Source: CAD feature listing. Evaluate the final solid. Frame: model axes, mm. Face numbers are marked on the shaded views. A direction names the side the tool comes from. Give positions to 0.01 mm unless a question says otherwise; leave off trailing zeros. Loops run counter-clockwise (first coordinate to the right, second up) from the corner with the lowest first, then second, coordinate; pieces in that order, holes last. Notation, with made-up numbers: M 75.25,23 L 120.25,23 A22 ccw 120.25,43 Z; hole C -38,89 d11. An arc over 180 degrees is marked long. Answer in a Markdown table with one row per item.
```python
from build123d import *

# Parameters (mm, degrees)
SKETCH2_W             = 20.32
SKETCH2_H             = 7.62
SKETCH2_R             = 1.905
BOSS_EXTRUDE1_DEPTH   = 12.7
BOSS_EXTRUDE1_2_DEPTH = 12.7
SKETCH4_W             = 3.81
SKETCH4_H             = 55.88
BOSS_EXTRUDE2_DEPTH   = 28.702
SKETCH5_W             = 27.94
SKETCH5_H             = 55.88
BOSS_EXTRUDE3_DEPTH   = 7.62
SKETCH6_R             = 10.922
BOSS_EXTRUDE6_DEPTH   = 55.88
SKETCH10_W            = 20.32
SKETCH10_H            = 16.002
BOSS_EXTRUDE7_DEPTH   = 7.62
SKETCH11_W            = 20.32
SKETCH11_H            = 16.002
BOSS_EXTRUDE8_DEPTH   = 7.62
SKETCH12_R            = 10.922
BOSS_EXTRUDE9_DEPTH   = 19.05
SKETCH14_R            = 2.921
BOSS_EXTRUDE10_DEPTH  = 74.93
SKETCH17_R            = 5.08
CUT_EXTRUDE3_DEPTH    = 32.766
SKETCH18_W            = 6.35
SKETCH18_H            = 7.62
CUT_EXTRUDE4_DEPTH    = 28.702


with BuildPart() as part:
    # Sketch2 → Boss-Extrude1 (new body)
    with BuildSketch(Plane.XY):
        with Locations((0, 24.13)):
            Rectangle(SKETCH2_W, SKETCH2_H)
        with Locations((4.699, 24.13)):
            Circle(SKETCH2_R, mode=Mode.SUBTRACT)
        with Locations((-4.699, 24.13)):
            Circle(SKETCH2_R, mode=Mode.SUBTRACT)
    extrude(amount=BOSS_EXTRUDE1_DEPTH)



with BuildPart() as body_2:
    # Sketch2 → Boss-Extrude1 2 (new body)
    with BuildSketch(Plane.XY):
        with Locations((0, -24.13)):
            Rectangle(SKETCH2_W, SKETCH2_H)
        with Locations((-4.699, -24.13)):
            Circle(SKETCH2_R, mode=Mode.SUBTRACT)
        with Locations((4.699, -24.13)):
            Circle(SKETCH2_R, mode=Mode.SUBTRACT)
    extrude(amount=BOSS_EXTRUDE1_2_DEPTH)


with BuildPart() as part_1:
    add(part.part)

    add(body_2.part)  # Boss-Extrude2 merges body 2
    # Sketch4 → Boss-Extrude2 (add)
    with BuildSketch(Plane.XY.offset(12.7)):
        with Locations((-12.065, 0)):
            Rectangle(SKETCH4_W, SKETCH4_H)
        with Locations((12.065, 0)):
            Rectangle(SKETCH4_W, SKETCH4_H)
    extrude(amount=-BOSS_EXTRUDE2_DEPTH)

    # Sketch5 → Boss-Extrude3 (add)
    with BuildSketch(Plane(origin=(0, 0, -16.002), x_dir=(-1, 0, 0), z_dir=(0, 0, -1))):
        Rectangle(SKETCH5_W, SKETCH5_H)
    extrude(amount=BOSS_EXTRUDE3_DEPTH)

    # Sketch6 → Boss-Extrude6 (add)
    with BuildSketch(Plane(origin=(0, 27.94, 0), x_dir=(1, 0, 0), z_dir=(0, 1, 0))):
        with BuildLine():
            Line((8.710385525, 23.622), (13.97, 23.622))
            Line((13.97, 23.622), (13.97, 34.544))
            ThreePointArc((13.97, 34.544), (0, 48.514), (-13.97, 34.544))
            Line((-13.97, 34.544), (-13.97, 23.622))
            Line((-13.97, 23.622), (-8.710385525, 23.622))
            ThreePointArc((-8.710385525, 23.622), (0, 20.574), (8.710385525, 23.622))
        make_face()
        with Locations((0, 34.544)):
            Circle(SKETCH6_R, mode=Mode.SUBTRACT)
    extrude(amount=-BOSS_EXTRUDE6_DEPTH)

    # Sketch10 → Boss-Extrude7 (add)
    with BuildSketch(Plane(origin=(0, 27.94, 0), x_dir=(1, 0, 0), z_dir=(0, 1, 0))):
        with Locations((0, 8.001)):
            Rectangle(SKETCH10_W, SKETCH10_H)
    extrude(amount=-BOSS_EXTRUDE7_DEPTH)

    # Sketch11 → Boss-Extrude8 (add)
    with BuildSketch(Plane.XZ.offset(27.94)):
        with Locations((0, -8.001)):
            Rectangle(SKETCH11_W, SKETCH11_H)
    extrude(amount=-BOSS_EXTRUDE8_DEPTH)

    # Sketch12 → Boss-Extrude9 (add)
    with BuildSketch(Plane(origin=(0, 27.94, 0), x_dir=(1, 0, 0), z_dir=(0, 1, 0))):
        Polygon((-13.97, -12.7), (-13.97, -39.878), (-5.207, -39.878), (-5.207, -34.925), (-10.287, -34.925), (-10.287, -29.591), (10.287, -29.591), (10.287, -34.925), (5.207, -34.925), (5.207, -39.878), (13.97, -39.878), (13.97, -12.7), align=None)
        with BuildLine():
            Line((13.97, -12.7), (13.97, 34.544))
            ThreePointArc((13.97, 34.544), (0, 48.514), (-13.97, 34.544))
            Line((-13.97, 34.544), (-13.97, -12.7))
            Line((-13.97, -12.7), (13.97, -12.7))
        make_face()
        with Locations((0, 34.544)):
            Circle(SKETCH12_R, mode=Mode.SUBTRACT)
    extrude(amount=BOSS_EXTRUDE9_DEPTH)

    # Sketch14 → Boss-Extrude10 (add)
    with BuildSketch(Plane(origin=(0, 46.99, 0), x_dir=(1, 0, 0), z_dir=(0, 1, 0))):
        with BuildLine():
            Line((21.132926123, 39.011999157), (6.635812906, 46.837367605))
            ThreePointArc((6.635812906, 46.837367605), (11.997149793, 41.701464415), (13.97, 34.544))
            Line((13.97, 34.544), (13.97, 26.397222721))
            Line((13.97, 26.397222721), (13.97, 23.366509606))
            ThreePointArc((13.97, 23.366509606), (14.856612526, 25.442827777), (16.555367234, 26.929909268))
            Line((16.555367234, 26.929909268), (21.132926123, 29.400820847))
            ThreePointArc((21.132926123, 29.400820847), (23.999926533, 34.206410002), (21.132926123, 39.011999157))
        make_face()
        with Locations((18.538926533, 34.206410002)):
            Circle(SKETCH14_R, mode=Mode.SUBTRACT)
    extrude(amount=-BOSS_EXTRUDE10_DEPTH)

    # Sketch17 → Cut-Extrude3 (cut)
    with BuildSketch(Plane(origin=(0, 0, -48.514), x_dir=(-1, 0, 0), z_dir=(0, 0, -1))):
        with Locations((0, 36.83)):
            Circle(SKETCH17_R)
    extrude(amount=-CUT_EXTRUDE3_DEPTH, mode=Mode.SUBTRACT)

    # Sketch18 → Cut-Extrude4 (cut)
    with BuildSketch(Plane.XY.offset(12.7)):
        with Locations((0, -24.13)):
            Rectangle(SKETCH18_W, SKETCH18_H)
    extrude(amount=-CUT_EXTRUDE4_DEPTH, mode=Mode.SUBTRACT)


solid = part_1.part
```
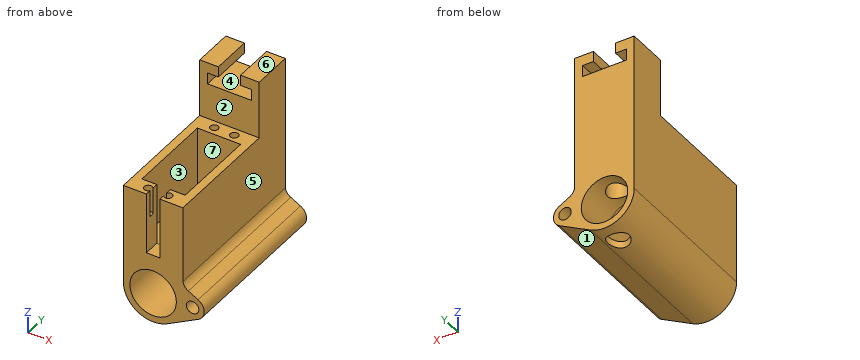
Q1. Section query B-B (z = -43). Output: boundary loops of the cut face in (x, y).
Values follow:
| item | result |
|---|---|
| outline | M -11.12,-27.94 L -6.91,-27.94 L -6.91,46.99 L -11.12,46.99 Z; M 6.91,-27.94 L 13.74,-27.94 L 13.74,46.99 L 6.91,46.99 Z |
Q2. Section query D-D (y = 13). Output: boundary loops of the cut face in (x, z), plus the area to 3 significant figures.
Values follow:
| item | result |
|---|---|
| outline | M -13.97,-34.54 A13.97 ccw 6.64,-46.84 L 21.13,-39.01 A5.46 ccw 21.13,-29.4 L 16.56,-26.93 A5.08 cw 13.97,-23.37 L 13.97,12.7 L 10.16,12.7 L 10.16,-16 L -10.16,-16 L -10.16,12.7 L -13.97,12.7 Z; hole C 0,-34.54 d21.84; hole C 18.54,-34.21 d5.84 |
| area | 771 mm^2 |
Q3. Reachability of the marked faces 5, 6 and 7 from +Z, -Z, +X, -X, +Y, -Y: full face, straight path, thin tool, end or side. Return the list, or none.
Values follow:
| item | result |
|---|---|
| face 5 | +Z, +X, +Y, -Y |
| face 6 | +Z, +X, -X, +Y, -Y |
| face 7 | +Z |
Q4. Contact query for flat-ended pins moving along their axis: pin 1 Ø2.5 at (x, y) = (-8.5, 39) entering from -Z; pin 2 Ø1 at (y, z) = (33, 21) entering from +X; pin 3 Ø1.7 at (x, y) = (5, -25) entering from +Z; pin 4 Ø19.5 at (x, z) = (0, -34.544) entering from +Y. Output: stop coordinate, or through.
Values follow:
| item | result |
|---|---|
| pin 1 | z = -46.49 |
| pin 2 | x = 13.97 |
| pin 3 | z = 0 |
| pin 4 | through |
Q5. Ray query, probe 1 along X at (y, z) = (24, 6); probe 2 along Y at (x, z) = (4.5, 10); probe 3 along Z at (x, y) = (0, -5). Return the intervals inside material, ascending. Write a range as from..to.
Values follow:
| item | result |
|---|---|
| probe 1 | -13.97..-6.6, -2.8..2.8, 6.6..13.97 |
| probe 2 | -27.94..-26.02, -22.24..-20.32, 20.32..22.24, 26.02..46.99 |
| probe 3 | -48.51..-45.47, -23.62..-16 |
Q6. Mould query, pull axis X, two halves, no side actions, for the marked faces 1, 2, 3 and 4. Classes: +X half, -X half, draft (parallel to the pull), parting line (faces both ways), or undercut.
Values follow:
| item | result |
|---|---|
| face 1 | +X half |
| face 2 | draft |
| face 3 | undercut |
| face 4 | undercut |
Q7. Section query C-C (z = 9). Output: boundary loops of the cut face in (x, y) (3 decimals), plus the area to 3 significant figures.
Values follow:
| item | result |
|---|---|
| outline | M -13.97,-27.94 L -3.175,-27.94 L -3.175,-25.273 A1.905 cw long -3.175,-22.987 L -3.175,-20.32 L -10.16,-20.32 L -10.16,20.32 L 10.16,20.32 L 10.16,-20.32 L 3.175,-20.32 L 3.175,-22.987 A1.905 cw long 3.175,-25.273 L 3.175,-27.94 L 13.97,-27.94 L 13.97,46.99 L -13.97,46.99 Z; hole C -4.699,24.13 d3.81; hole C 4.699,24.13 d3.81 |
| area | 1,170 mm^2 |
Q8. Section query A-A (x = 0). Output: boundary loops of the cut face in (y, z).
Values follow:
| item | result |
|---|---|
| outline | M -27.94,-48.51 L 31.75,-48.51 L 31.75,-45.47 L -27.94,-45.47 Z; M -27.94,-23.62 L 31.75,-23.62 L 31.75,-15.75 L 41.91,-15.75 L 41.91,-23.62 L 46.99,-23.62 L 46.99,29.59 L 27.94,29.59 L 27.94,12.7 L 20.32,12.7 L 20.32,-16 L -27.94,-16 Z; M 41.91,-48.51 L 46.99,-48.51 L 46.99,-45.47 L 41.91,-45.47 Z |
